Can you work these out from the model? Positions are in its coordinate system, mm. A direction names the side the tool comes from. Coordinates: 2 decimals unless noted, no trailing zeros. Order: outer loops, then holes, each group sorted by start corner. A loop starts at its lowest first (then second) coordinate and runs counter-clockwise, first axis right, second up. Notation, with made-up numbers: (83, 51) -> (117, 51) arc R5 ccw to (117, 59) -> close; hole circle Ø6 at (74.25, -13.75). An arc over 180 degrees is marked (long way). Answer in a Markdown table with one row per item. Add a question column.
1. Imagine slicing it at A-A on z = -2. Write out the boundary of the cut face in (x, y).
2. If I drill on line 1 along X through (y, z) = (0.5, 15.25); line 2 along X through (y, z) = (-11, -2.5); line 3 along Z through (x, y) = (8, 15.5), over which ranges is the centre line in solid material (lowest first)? Write a range as [from, to].
3. Will these pins go through, and if not, where does the flat tip stop? pin 1 (5 mm diameter, centred on y = -15.5, z = 9, fed in from -X); pin 2 (2 mm diameter, centred on y = 2, z = 16, fed in from +X); pin 3 (8 mm diameter, centred on x = 11.5, y = 2, fed in from +Z); pin 4 (2 mm diameter, centred on y = 15.5, z = -2.5, fed in from -X).
4. On a 3-axis mill with a long thin cutter (end or side, diameter ignored), from which of +Z, -Z, +X, -X, +Y, -Y can I reach the whole of each face in a straight line? I mean faces 1 (the face through (5, 12, -3)), 2 (the face through (0, -10.25, -3)), 3 (the face through (0, -13.75, -3)). Say none if no direction works.
5. We'd pull the mould along Y, two halves only. Please class faces 4 (the face through (0, 13.75, -3)), 5 (the face through (0, -14, 0)), 6 (the face through (0, 12, -6)): pulls with the +Y half, pulls with the -Y half, needs draft (parallel to the pull), parting line crosses it, or undercut.
from build123d import *

# Parameters (mm, degrees)
REVOLVE_1_ANGLE = 180
FILLET_1_R      = 5
FILLET_2_R      = 5
SKETCH_3_W      = 10
SKETCH_3_H      = 3.5
EXTRUDE_1_DEPTH = 6


with BuildPart() as part:
    # 草图1 → 旋转1 (revolve)
    with BuildSketch(Plane.XY):
        with BuildLine():
            Line((-15, 5), (15, 5))
            ThreePointArc((15, 5), (14.412847263, 11.739422714), (12.669081334, 18.275770872))
            ThreePointArc((12.669081334, 18.275770872), (0, 20), (-12.669081334, 18.275770872))
            ThreePointArc((-12.669081334, 18.275770872), (-14.412847263, 11.739422714), (-15, 5))
        make_face()
    revolve(axis=Axis((-17.5, 0, 0), (1, 0, 0)), revolution_arc=REVOLVE_1_ANGLE)

    # 圆角1
    fillet_1_edges = [part.edges().sort_by_distance(p)[0] for p in [
        (12.669081334, 0, 18.275770872),
        (-12.669081334, 0, 18.275770872),
    ]]
    fillet(fillet_1_edges, radius=FILLET_1_R)

    # 圆角2
    fillet_2_edges = [part.edges().sort_by_distance(p)[0] for p in [
        (-15, 0, 5),
        (15, 0, 5),
    ]]
    fillet(fillet_2_edges, radius=FILLET_2_R)

    # 草图3 → 凸台-拉伸1 (add)
    with BuildSketch(Plane(origin=(0, 0, 0), x_dir=(-1, 0, 0), z_dir=(0, 0, -1))):
        with Locations((0, 12)):
            Rectangle(SKETCH_3_W, SKETCH_3_H)
        with Locations((0, -12)):
            Rectangle(SKETCH_3_W, SKETCH_3_H)
    extrude(amount=EXTRUDE_1_DEPTH)


solid = part.part
Answers follow:
| question | item | result |
|---|---|---|
| 1 | outline | (-5, -13.75) -> (5, -13.75) -> (5, -10.25) -> (-5, -10.25) -> close; (-5, 10.25) -> (5, 10.25) -> (5, 13.75) -> (-5, 13.75) -> close |
| 2 | line 1 | x = [-13.63, 13.63] |
| 2 | line 2 | x = [-5, 5] |
| 2 | line 3 | z = [0, 11.53] |
| 3 | pin 1 | stops at x = -13.58 |
| 3 | pin 2 | stops at x = 13.66 |
| 3 | pin 3 | stops at z = 19.36 |
| 3 | pin 4 | passes through |
| 4 | face 1 | -Z, +X, +Y, -Y |
| 4 | face 2 | -Z, +X, -X |
| 4 | face 3 | -Z, +X, -X, -Y |
| 5 | face 4 | pulls with the +Y half |
| 5 | face 5 | undercut |
| 5 | face 6 | needs draft |
